Work out the finished part from the listing and answer in its coordinate system (mm). A direction names the side the tool comes from. Round coordinates to 2 decimals unless told otherwise and drop trailing zeros. Order: outer loops, then holes, each group sorted by start corner. A loop starts at its lowest first (then second) coordinate and runs counter-clockwise, first axis right, second up. Notation, with made-up numbers: M 31.5,32.5 L 80.5,32.5 A20 ccw 80.5,69.5 Z; hole C 53.25,-30 d8. An arc over 180 degrees is marked long. Return JSON: item names as keys, results as strings.
from build123d import *

# Parameters (mm, degrees)
BASE_FLANGE1_DEPTH = 10
FILLET1_R          = 3
SKETCH6_R          = 1.5
CUT_EXTRUDE1_DEPTH = 18.549928775
SKETCH11_R         = 1
CUT_EXTRUDE2_DEPTH = 2


# Sheet-metal steps are written as plain solids
with BuildPart() as part:
    # Sketch1 → Base-Flange1 (new, symmetric)
    with BuildSketch(Plane.XY):
        with BuildLine():
            Line((-12, 0), (-0.75, 0))
            ThreePointArc((-0.75, 0), (-0.219669914, 0.219669914), (0, 0.75))
            Line((0, 0.75), (0, 8))
            Line((0, 8), (2, 8))
            Line((2, 8), (2, 0.75))
            ThreePointArc((2, 0.75), (1.194543648, -1.194543648), (-0.75, -2))
            Line((-0.75, -2), (-12, -2))
            Line((-12, -2), (-12, 0))
        make_face()
    extrude(amount=BASE_FLANGE1_DEPTH, both=True)

    # Fillet1
    fillet1_edges = [part.edges().sort_by_distance(p)[0] for p in [
        (-12, -1, 10),
        (-12, -1, -10),
        (1, 8, 10),
        (1, 8, -10),
    ]]
    fillet(fillet1_edges, radius=FILLET1_R)

    # Sketch6 → Cut-Extrude1 (cut, through all)
    with BuildSketch(Plane(origin=(0, 0, 0), x_dir=(1, 0, 0), z_dir=(0, 1, 0))):
        with Locations(Location((-9, 6, 0), (0, 0, 270))):
            Circle(SKETCH6_R)
        with Locations(Location((-9, -6, 0), (0, 0, 90))):
            Circle(SKETCH6_R)
    extrude(amount=-CUT_EXTRUDE1_DEPTH, mode=Mode.SUBTRACT)

    # Sketch11 → Cut-Extrude2 (cut)
    with BuildSketch(Plane.ZY):
        with Locations((6, 4)):
            Circle(SKETCH11_R)
        with Locations((-6, 4)):
            Circle(SKETCH11_R)
    extrude(amount=-CUT_EXTRUDE2_DEPTH, mode=Mode.SUBTRACT)


solid = part.part
Item 1: Consider line 1 along Y through (x, z) = (-9.25, -2); line 2 along X through (y, z) = (2, 7.75); line 3 along Y through (x, z) = (0.45, 6). Determine where each line is inside the solid, lowest interval first. Write a range as [from, to].
Output:
{"line 1": "y = [-2, 0]", "line 2": "x = [0, 2]", "line 3": "y = [-1.72, 3], [5, 8]"}
Item 2: Which of the six approach directions +Z, -Z, +X, -X, +Y, -Y give full straight-line access (tool end or side, diameter ignored) to faces 1 (the flat face through (-2, -1, 10)), 2 (the flat face through (0, 4, 0))?
Output:
{"face 1": "+Z, +X, -X, +Y, -Y", "face 2": "+Z, -Z, -X, +Y"}
Item 3: The mould has two halves that part along Y. Classify faces 3 (the cylindrical face through (1.01, 7.1, 9.14)), 4 (the cylindrical face through (0.986, 4.676, -6.737)), 5 (the cylindrical face through (-7.536, -0.986, 6.325)), 6 (the cylindrical face through (1.22, -1.17, 0.14)): pulls with the +Y half, pulls with the -Y half, needs draft (parallel to the pull), parting line crosses it, or undercut.
Output:
{"face 3": "pulls with the +Y half", "face 4": "undercut", "face 5": "needs draft", "face 6": "pulls with the -Y half"}
Item 4: Find section A-A (z = 6). Determine the outline of the cut face in (x, y), plus the area to 3 significant figures.
Output:
{"outline": "M -12,-2 L -10.5,-2 L -10.5,0 L -12,0 Z; M -7.5,-2 L -0.75,-2 A2.75 ccw 2,0.75 L 2,3 L 0,3 L 0,0.75 A0.75 cw -0.75,0 L -7.5,0 Z; M 0,5 L 2,5 L 2,8 L 0,8 Z", "area": "32.5 mm^2"}
Item 5: Each of these flat-tipped pins is pushed along its axis until it touches: pin 1 (2 mm diameter, centred on y = 3, z = -3, fed in from -X); pin 2 (3.5 mm diameter, centred on x = -9, z = 6, fed in from +Y). Where does it stop, or does it pass through?
Output:
{"pin 1": "stops at x = 0", "pin 2": "stops at y = 0"}
Item 6: Find section B-B (y = 4). Determine the outline of the cut face in (x, z).
Output:
{"outline": "M 0,-10 L 2,-10 L 2,-7 L 0,-7 Z; M 0,-5 L 2,-5 L 2,5 L 0,5 Z; M 0,7 L 2,7 L 2,10 L 0,10 Z"}
Item 7: Find section D-D (y = -0.5). Determine the outline of the cut face in (x, z).
Output:
{"outline": "M -12,-7 A3 ccw -9,-10 L 1.7,-10 L 1.7,10 L -9,10 A3 ccw -12,7 Z; hole C -9,-6 d3; hole C -9,6 d3"}
Item 8: Find section C-C (z = -4). Determine the outline of the cut face in (x, y).
Output:
{"outline": "M -12,-2 L -0.75,-2 A2.75 ccw 2,0.75 L 2,8 L 0,8 L 0,0.75 A0.75 cw -0.75,0 L -12,0 Z"}
